```python
from build123d import *

# Parameters (mm, degrees)
BOSS_EXTRUDE1_DEPTH                                  = 16
CSK_FOR_M5_HEX_SOCKET_COUNTERSUNK_CAP_SC_D           = 6.6
CSK_FOR_M5_HEX_SOCKET_COUNTERSUNK_CAP_SC_CSINK_D     = 7
CSK_FOR_M5_HEX_SOCKET_COUNTERSUNK_CAP_SC_CSINK_ANGLE = 90
CBORE_FOR_M4_HEX_SOCKET_HEAD_CAP_SCREW1_D            = 4.5
CBORE_FOR_M4_HEX_SOCKET_HEAD_CAP_SCREW1_CBORE_D      = 8
CBORE_FOR_M4_HEX_SOCKET_HEAD_CAP_SCREW1_CBORE_DEPTH  = 4.4


with BuildPart() as part:
    # Sketch1 → Boss-Extrude1 (new body)
    with BuildSketch(Plane.XY):
        with BuildLine():
            Line((24, 0), (-24, 0))
            Line((-24, 0), (-24, 7))
            ThreePointArc((-24, 7), (-23.707106781, 7.707106781), (-23, 8))
            Line((-23, 8), (-12.5, 8))
            Line((-12.5, 8), (-12.5, 42))
            ThreePointArc((-12.5, 42), (-11.914213562, 43.414213562), (-10.5, 44))
            Line((-10.5, 44), (-2.731683137, 44))
            Line((-2.731683137, 44), (-2.731683137, 34.519169318))
            ThreePointArc((-2.731683137, 34.519169318), (0, 19), (2.731683137, 34.519169318))
            Line((2.731683137, 34.519169318), (2.731683137, 44))
            Line((2.731683137, 44), (10.5, 44))
            ThreePointArc((10.5, 44), (11.914213562, 43.414213562), (12.5, 42))
            Line((12.5, 42), (12.5, 8))
            Line((12.5, 8), (23, 8))
            ThreePointArc((23, 8), (23.707106781, 7.707106781), (24, 7))
            Line((24, 7), (24, 0))
        make_face()
    extrude(amount=BOSS_EXTRUDE1_DEPTH)

    # CSK for M5 Hex Socket Countersunk Cap Screw1 (through all)
    with Locations(Plane(origin=(-19, 8, 8), x_dir=(0, 0, 1), z_dir=(0, 1, 0))):
        with Locations((0, 0), (0, 38)):
            CounterSinkHole(CSK_FOR_M5_HEX_SOCKET_COUNTERSUNK_CAP_SC_D / 2, CSK_FOR_M5_HEX_SOCKET_COUNTERSUNK_CAP_SC_CSINK_D / 2, counter_sink_angle=CSK_FOR_M5_HEX_SOCKET_COUNTERSUNK_CAP_SC_CSINK_ANGLE)

    # CBORE for M4 Hex Socket Head Cap Screw1 (through all)
    with Locations(Plane(origin=(12.5, 38, 8), x_dir=(0, 0, 1), z_dir=(1, 0, 0))):
        with Locations((0, 0)):
            CounterBoreHole(CBORE_FOR_M4_HEX_SOCKET_HEAD_CAP_SCREW1_D / 2, CBORE_FOR_M4_HEX_SOCKET_HEAD_CAP_SCREW1_CBORE_D / 2, CBORE_FOR_M4_HEX_SOCKET_HEAD_CAP_SCREW1_CBORE_DEPTH)


solid = part.part
```
Verification items for the finished model (mm, model axes). A direction names the side the tool comes from. Round coordinates to 2 decimals unless told otherwise and drop trailing zeros. Write each loop counter-clockwise with the first axis right and the second up, starting at its lowest first coordinate (ties: lowest second). Pieces come first, ordered by that corner, then holes.
1. Section check A-A on y = 38. Enter the section's corners in (x, z), plus the area to 3 significant figures.
2. Gauge pin test, flat ends, axial feed: P1, Ø2.5, axis at y = 38, z = 8, coming from the +X side (1 decimal); P2, Ø5, axis at x = 19.5, z = 6.5, coming from the +Y side; P3, Ø5, axis at y = 38, z = 8, coming from the -X side; P4, Ø4, axis at y = 11.5, z = 11.5, coming from the +X side. Record the tip position at first contact, or that the pin passes through.
3. Access from +Z, -Z, +X, -X, +Y, -Y to the whole of each face (thin tool, end or side, straight path). Record for faces 4 (the flat face through (2.732, 41, 8)), 5 (the flat face through (0, 0, 8)), 6 (the flat face through (8.1, 40, 10)), 7 (the flat face through (-12.5, 25, 8)).
4. Section check B-B on x = 19. Enter the section's corners in (y, z), plus the area to 3 significant figures.
5. Scan lines: L1, parallel to X at y = 4.5, z = 8; L2, parallel to X at y = 42, z = 11.5; L3, parallel to Z at x = -19, y = 4. Record each from-to range of solid material in increasing order.
6. Section check D-D on y = 23.5. Enter the section's corners in (x, z), plus the area to 3 significant figures.
7. Draft check along Z on faces 1 (the flat face through (0, 17, 0)), 2 (the cylindrical face through (-21.008, 3.845, 10.619)), 3 (the flat face through (15, 8, 8)). Enter one of: +Z half, -Z half, draft (parallel to the pull), parting line (faces both ways), or undercut.
8. Section check C-C on x = -3.5. Enter the section's corners in (y, z), plus the area to 3 significant figures.
Answer:
1. outline: (-12.5, 0) - (-2.73, 0) - (-2.73, 5.75) - (-12.5, 5.75) - close; (-12.5, 10.25) - (-2.73, 10.25) - (-2.73, 16) - (-12.5, 16) - close; (2.73, 0) - (12.5, 0) - (12.5, 4) - (8.1, 4) - (8.1, 5.75) - (2.73, 5.75) - close; (2.73, 10.25) - (8.1, 10.25) - (8.1, 12) - (12.5, 12) - (12.5, 16) - (2.73, 16) - close
1. area: 209 mm2
2. P1: passes through
2. P2: stops at y = 8
2. P3: stops at x = -12.5
2. P4: stops at x = 12.5
3. face 4: +Z, -Z, +Y
3. face 5: +Z, -Z, +X, -X, -Y
3. face 6: +X
3. face 7: +Z, -Z, -X, +Y
4. outline: (0, 0) - (8, 0) - (8, 4.5) - (7.8, 4.7) - (0, 4.7) - close; (0, 11.3) - (7.8, 11.3) - (8, 11.5) - (8, 16) - (0, 16) - close
4. area: 75.2 mm2
5. L1: x = -24 to -22.3, -15.7 to 15.7, 22.3 to 24
5. L2: x = -12.5 to -2.73, 2.73 to 12.5
5. L3: z = 0 to 4.7, 11.3 to 16
6. outline: (-12.5, 0) - (-7.19, 0) - (-7.19, 16) - (-12.5, 16) - close; (7.19, 0) - (12.5, 0) - (12.5, 16) - (7.19, 16) - close
6. area: 170 mm2
7. face 1: -Z half
7. face 2: undercut
7. face 3: draft
8. outline: (0, 0) - (19.81, 0) - (19.81, 16) - (0, 16) - close; (34.19, 0) - (44, 0) - (44, 16) - (34.19, 16) - close; hole circle Ø4.5 at (38, 8)
8. area: 458 mm2
